```python
from build123d import *

# Parameters (mm, degrees)
F0_W     = 50.8
F0_H     = 76.2
F1_DEPTH = 6.35
F2_D     = 10.3124
F3_R     = 14.2875
F4_DEPTH = 19.05
F5_R     = 9.525
F6_DEPTH = 26.9875


with BuildPart() as f1:
    # F0 (on Front) → F1 (new body)
    with BuildSketch(Plane.XZ):
        Rectangle(F0_W, F0_H)
    extrude(amount=F1_DEPTH)

    # F2 (through all)
    with Locations(Plane(origin=(0, 0, 0), x_dir=(1, 0, 0), z_dir=(0, 1, 0))):
        with Locations((0, -28.575), (0, 28.575)):
            Hole(F2_D / 2)

    # F3 (on face) → F4 (join)
    with BuildSketch(Plane.XZ.offset(6.35)):
        Circle(F3_R)
    extrude(amount=F4_DEPTH)

    # F5 (on face) → F6 (join)
    with BuildSketch(Plane.XZ.offset(25.4)):
        Circle(F5_R)
    extrude(amount=F6_DEPTH)


solid = f1.part
```
Can you work these out from the model? Positions are in its coordinate system, mm. A direction names the side the tool comes from. Coordinates: 2 decimals unless noted, no trailing zeros. Loops run counter-clockwise (first coordinate to the right, second up) from the corner with the lowest first, then second, coordinate; pieces in that order, holes last. Notation, with made-up numbers: (-19, 86) - (-6, 86) arc R29 ccw to (-6, 121) - close; hole circle Ø7 at (51.5, -7.5). An arc over 180 degrees is marked (long way). Use a Markdown table: item, result.
Item 1: I want a section at D-D on y = -24.5. Please give me the cut outline in (x, z) (1 decimal), and give its area (3 significant figures).
Numbers:
| item | result |
|---|---|
| outline | circle Ø28.6 at (0, 0) |
| area | 641 mm2 |
Item 2: If I drill on probe 1 along Z at (x, y) = (0, -2.75); probe 2 along Y at (x, z) = (-2, -22); probe 3 along Z at (x, y) = (8, -38), over which ranges is the centre line in solid material (lowest first)? Write a range as from..to.
Numbers:
| item | result |
|---|---|
| probe 1 | z = -38.1..-33.73, -23.42..23.42, 33.73..38.1 |
| probe 2 | y = -6.35..0 |
| probe 3 | z = -5.17..5.17 |
Item 3: We'd pull the mould along X, two halves only. Please class faces 3 (the face through (0, -52.388, 0)), 4 (the face through (3.8, -3.22, -32.06)), 5 (the face through (25.4, -3, -1)), 6 (the face through (0.671, -3.219, 23.463)): released by +X, released by -X, zero draft, split by the parting line, or undercut.
Numbers:
| item | result |
|---|---|
| face 3 | zero draft |
| face 4 | undercut |
| face 5 | released by +X |
| face 6 | undercut |
Item 4: Will these pins go through, and if not, where does the flat tip stop? pin 1 (10 mm diameter, centred on x = 18, z = -14, fed in from -Y); pin 2 (4 mm diameter, centred on x = -2, y = -19, fed in from -Z); pin 3 (8 mm diameter, centred on x = 14.5, y = -45.5, fed in from -Z); pin 4 (2 mm diameter, centred on x = 14, y = -18, fed in from -Z).
Numbers:
| item | result |
|---|---|
| pin 1 | stops at y = -6.35 |
| pin 2 | stops at z = -14.29 |
| pin 3 | passes through |
| pin 4 | stops at z = -5.93 |
Item 5: I want a section at B-B on z = -31.5. Please give me the cut outline in (x, y), and give its area (3 significant figures).
Numbers:
| item | result |
|---|---|
| outline | (-25.4, -6.35) - (-4.25, -6.35) - (-4.25, 0) - (-25.4, 0) - close; (4.25, -6.35) - (25.4, -6.35) - (25.4, 0) - (4.25, 0) - close |
| area | 269 mm2 |
Item 6: For faces 1 (the face through (3, -25.4, -9.3)), 2 (the face through (0, -3, -38.1)), which set-ups out of +Z, -Z, +X, -X, +Y, -Y let a thin tool reach every point of the face, with its end or its side?
Numbers:
| item | result |
|---|---|
| face 1 | -Y |
| face 2 | -Z, +X, -X, +Y, -Y |
Item 7: I want a section at A-A on x = 0. Give the number of separate pieces and of enclosed holes in the cut face, and give its area (3 significant figures).
Numbers:
| item | result |
|---|---|
| separate pieces | 3 |
| enclosed holes | 0 |
| area | 1,410 mm2 |
